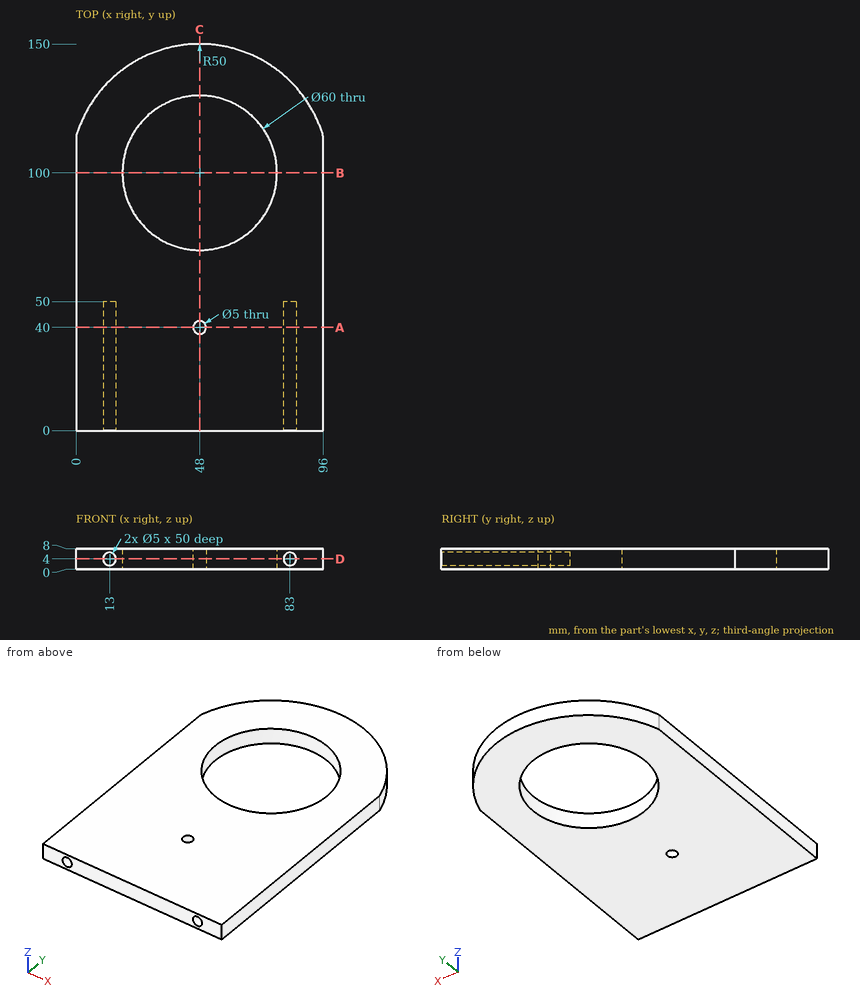
Source: three-view drawing plus pictorial views. Frame: mm from the lowest corner of the part. Round coordinates to 2 decimals unless told otherwise and drop trailing zeros. Loops run counter-clockwise (first coordinate to the right, second up) from the corner with the lowest first, then second, coordinate; pieces in that order, holes last. Notation, with made-up numbers: M 79,-35.75 L 118,-35.75 A12 ccw 118,-19.75 Z; hole C -19.5,76.25 d2. An arc over 180 degrees is marked long. Answer as CSV lines item,"result". Start each with the question number.
(1) Section C-C, the plane x = 48. Output: boundary loops of the cut face in (y, z).
(2) Section A-A, the plane y = 40. Output: boundary loops of the cut face in (x, z).
(3) First-contact query: pin 1 (1.5 mm diameter, centred on x = 73.5, z = 3, fed in from -Y); pin 2 (4 mm diameter, centred on x = 48, y = 40, fed in from +Z); pin 3 (4.5 mm diameter, centred on x = 13, z = 4, fed in from +Y); pin 4 (2.5 mm diameter, centred on x = 83, z = 3, fed in from -Y). Flat tips, straight axial feed; report the tip coordinate or a pass-through.
(4) Line query: line 1 (X direction, y = 18.5, z = 4); line 2 (Y direction, x = 48, z = 5); line 3 (X direction, y = 17, z = 3). Output: solid intervals per line, ascending. Write a range as [from, to].
(5) Section D-D, the plane z = 4. Output: boundary loops of the cut face in (x, y), plus the area to 3 significant figures.
(6) Section B-B, the plane y = 100. Output: boundary loops of the cut face in (x, z), plus the area to 3 significant figures.
Values found:
1,outline,"M 0,0 L 37.5,0 L 37.5,8 L 0,8 Z; M 42.5,0 L 70,0 L 70,8 L 42.5,8 Z; M 130,0 L 150,0 L 150,8 L 130,8 Z"
2,outline,"M 0,0 L 45.5,0 L 45.5,8 L 0,8 Z; M 50.5,0 L 96,0 L 96,8 L 50.5,8 Z; hole C 13,4 d5; hole C 83,4 d5"
3,pin 1,"stops at y = 0"
3,pin 2,"passes through"
3,pin 3,"stops at y = 137.78"
3,pin 4,"stops at y = 50"
4,line 1,"x = [0, 10.5], [15.5, 80.5], [85.5, 96]"
4,line 2,"y = [0, 37.5], [42.5, 70], [130, 150]"
4,line 3,"x = [0, 10.71], [15.29, 80.71], [85.29, 96]"
5,outline,"M 0,0 L 10.5,0 L 10.5,50 L 15.5,50 L 15.5,0 L 80.5,0 L 80.5,50 L 85.5,50 L 85.5,0 L 96,0 L 96,114 A50 ccw 0,114 Z; hole C 48,100 d60; hole C 48,40 d5"
5,area,"10,100 mm²"
6,outline,"M 0,0 L 18,0 L 18,8 L 0,8 Z; M 78,0 L 96,0 L 96,8 L 78,8 Z"
6,area,"288 mm²"
